from build123d import *

# Parameters (mm, degrees)
SKETCH1_W           = 36.83
SKETCH1_H           = 20.32
BOSS_EXTRUDE1_DEPTH = 18.796
FILLET1_R           = 3.175
BOSS_EXTRUDE2_DEPTH = 25.908
BOSS_EXTRUDE3_DEPTH = 8.382
SKETCH4_R           = 1.5875
CUT_EXTRUDE1_DEPTH  = 19.796
BOSS_EXTRUDE4_START = -7.112
SKETCH5_W           = 4.826
SKETCH5_H           = 4.826
SKETCH5_R           = 1.5875
BOSS_EXTRUDE4_DEPTH = 2.54
FILLET2_R           = 0.635
BOSS_EXTRUDE5_DEPTH = 2.54
BOSS_EXTRUDE6_DEPTH = 4.064
FILLET3_R           = 1.27
SKETCH8_R           = 1.905
BOSS_EXTRUDE7_DEPTH = 1.524
FILLET4_R           = 0.635


with BuildPart() as part:
    # Sketch1 → Boss-Extrude1 (new body)
    with BuildSketch(Plane.XY):
        with Locations((18.415, 0)):
            Rectangle(SKETCH1_W, SKETCH1_H)
    extrude(amount=BOSS_EXTRUDE1_DEPTH)

    # Fillet1
    fillet1_edges = [part.edges().sort_by_distance(p)[0] for p in [
        (36.83, 10.16, 9.398),
        (36.83, -10.16, 9.398),
    ]]
    fillet(fillet1_edges, radius=FILLET1_R)

    # Sketch2 → Boss-Extrude2 (add)
    with BuildSketch(Plane.ZY):
        with BuildLine():
            ThreePointArc((3.96514897, 10.16), (1.809887501, 8.860648824), (0, 7.112))
            Line((0, 7.112), (0, -7.112))
            ThreePointArc((0, -7.112), (1.809887501, -8.860648824), (3.96514897, -10.16))
            Line((3.96514897, -10.16), (13.276942782, -10.16))
            ThreePointArc((13.276942782, -10.16), (15.61217315, -8.719352926), (17.526, -6.753130241))
            Line((17.526, -6.753130241), (17.526, 6.753130241))
            ThreePointArc((17.526, 6.753130241), (15.61217315, 8.719352926), (13.276942782, 10.16))
            Line((13.276942782, 10.16), (3.96514897, 10.16))
        make_face()
    extrude(amount=BOSS_EXTRUDE2_DEPTH)

    # Sketch3 → Boss-Extrude3 (add)
    with BuildSketch(Plane.XY.offset(18.796)):
        with BuildLine():
            Line((24.267261803, 2.273434446), (23.149675051, -1.177980315))
            ThreePointArc((23.149675051, -1.177980315), (24.617532764, -2.416473676), (26.532738197, -2.273434446))
            Line((26.532738197, -2.273434446), (27.650324949, 1.177980315))
            ThreePointArc((27.650324949, 1.177980315), (26.182467236, 2.416473676), (24.267261803, 2.273434446))
        make_face()
    extrude(amount=BOSS_EXTRUDE3_DEPTH)

    # Sketch4 → Cut-Extrude1 (cut, through all)
    with BuildSketch(Plane.XY.offset(18.796)):
        with Locations((5.588, 7.8105)):
            Circle(SKETCH4_R)
        with Locations((5.588, -7.8105)):
            Circle(SKETCH4_R)
    extrude(amount=-CUT_EXTRUDE1_DEPTH, mode=Mode.SUBTRACT)

    # Sketch5 → Boss-Extrude4 (add)
    with BuildSketch(Plane(origin=(0, 0, 0), x_dir=(-1, 0, 0), z_dir=(0, 0, -1)).offset(BOSS_EXTRUDE4_START)):
        with Locations((-39.243, 0)):
            Rectangle(SKETCH5_W, SKETCH5_H)
        with Locations((-39.243, 0)):
            Circle(SKETCH5_R, mode=Mode.SUBTRACT)
    extrude(amount=-BOSS_EXTRUDE4_DEPTH)

    # Fillet2
    fillet2_edges = [part.edges().sort_by_distance(p)[0] for p in [
        (41.656, 2.413, 8.382),
        (36.83, 2.413, 8.382),
        (36.83, -2.413, 8.382),
        (41.656, -2.413, 8.382),
    ]]
    fillet(fillet2_edges, radius=FILLET2_R)

    # Sketch6 → Boss-Extrude5 (add, symmetric)
    with BuildSketch(Plane(origin=(0, 0, 0), x_dir=(-1, 0, 0), z_dir=(0, -1, 0))):
        Polygon((4.430989114, -19.812), (6.716989114, -19.812), (6.716989114, -19.05), (7.478989114, -17.526), (4.430989114, -17.526), align=None)
        Polygon((6.716989114, 2.286), (6.716989114, 1.524), (7.478989114, 0), (4.430989114, 0), (4.430989114, 2.286), align=None)
    extrude(amount=BOSS_EXTRUDE5_DEPTH, both=True)

    # Sketch6<3> → Boss-Extrude6 (add, symmetric)
    with BuildSketch(Plane(origin=(0, 0, 0), x_dir=(-1, 0, 0), z_dir=(0, -1, 0))):
        Polygon((17.526, 0), (18.796, 1.27), (25.908, 1.27), (25.908, 0), align=None)
    extrude(amount=BOSS_EXTRUDE6_DEPTH, both=True)

    # Fillet3
    fillet3_edges = [part.edges().sort_by_distance(p)[0] for p in [
        (-25.908, 0, -1.27),
        (-18.796, 0, -1.27),
    ]]
    fillet(fillet3_edges, radius=FILLET3_R)

    # Sketch8 → Boss-Extrude7 (add)
    with BuildSketch(Plane.XY.offset(18.796)):
        with Locations((16.651010886, 0)):
            Circle(SKETCH8_R)
    extrude(amount=BOSS_EXTRUDE7_DEPTH)

    # Fillet4
    fillet4_edges = [part.edges().sort_by_distance(p)[0] for p in [
        (14.746010886, 0, 20.32),
    ]]
    fillet(fillet4_edges, radius=FILLET4_R)


solid = part.part
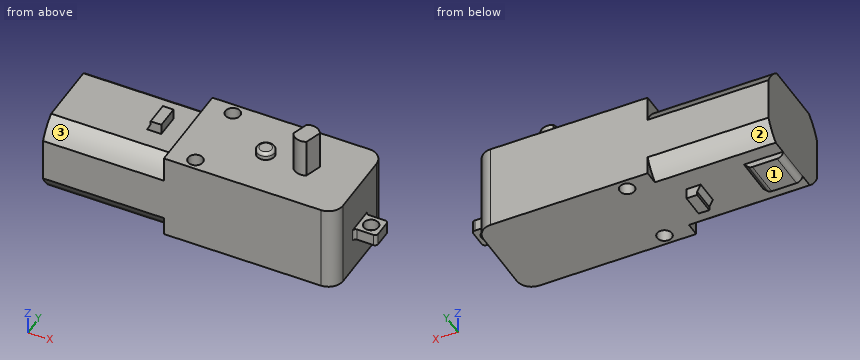
Here's how the part is built. I have some questions about the finished solid (model axes, mm). Face numbers are marked on the shaded views. A direction names the side the tool comes from. Coordinates: 2 decimals unless noted, no trailing zeros. Loops run counter-clockwise (first coordinate to the right, second up) from the corner with the lowest first, then second, coordinate; pieces in that order, holes last.
1. Imagine slicing it at D-D, the plane x = 36. Please give me the cut outline in (y, z).
2. I need wall thicknesses on L1, parallel to Z at x = 24, y = 6.5; L2, parallel to X at y = 1.5, z = 15.5; L3, parallel to Z at x = -0.5, y = -0.25. Which ranges of each line are inside material? Lowest first, please.
3. For P1, Ø2.5, axis at x = 40, y = -1.5, coming from the +Z side; P2, Ø2.5, axis at x = 39.243, y = 0, coming from the +Z side; P3, Ø1.1, axis at x = -5.5, z = -1, coming from the -Y side; P4, Ø5, axis at x = 5.59, y = -7.81, coming from the +Z side, each with a flat end and sliding along its axis, tell me the tip position at first contact or that it passes through.
4. Imagine slicing it at B-B, the plane x = 6. Please give me the cut outline in (y, z), and give its area (3 significant figures).
5. Imagine slicing it at A-A, the plane z = 5.75. Count the separate pieces of the cut face and the enclosed holes in it, and give its area (3 significant figures).
6. For the marked faces 1, 2 and 3, which set-ups out of +Z, -Z, +X, -X, +Y, -Y let a thin tool reach every point of the face, with its end or its side?
Taken from the geometry:
1. outline: (-9.13, 0) - (9.13, 0) - (9.13, 18.8) - (-9.13, 18.8) - close
2. L1: z = 0 to 18.8
2. L2: x = -25.91 to 36.83
2. L3: z = 0 to 17.53
3. P1: stops at z = 9.65
3. P2: passes through
3. P3: stops at y = -2.54
3. P4: stops at z = 18.8
4. outline: (-10.16, 0) - (-9.34, 0) - (-9.34, 18.8) - (-10.16, 18.8) - close; (-6.28, 0) - (6.28, 0) - (6.28, 18.8) - (-6.28, 18.8) - close; (9.34, 0) - (10.16, 0) - (10.16, 18.8) - (9.34, 18.8) - close
4. area: 267 mm2
5. separate pieces: 1
5. enclosed holes: 2
5. area: 1,250 mm2
6. face 1: -Z, -X, +Y, -Y
6. face 2: -Z, -X, +Y
6. face 3: +Z, -X, -Y
